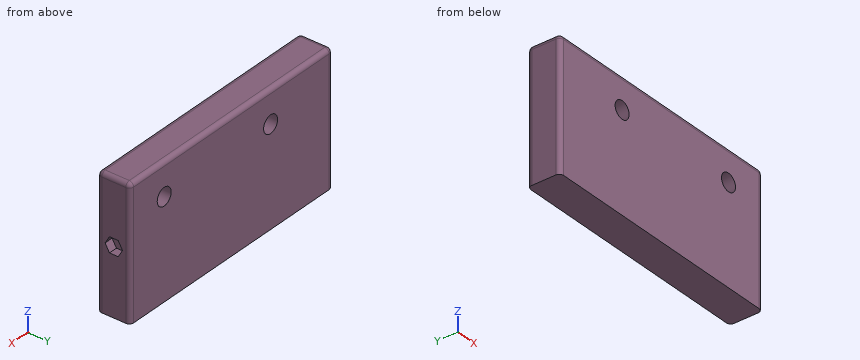
Solid Edge part; units mm, degrees
sketch "Sketch1" plane through (0, 0, 0) normal (1, 0, 0) x (0, 1, 0)
  line L0 (7.5, 30) -> (-7.5, 30)
  line L1 (-7.5, 30) -> (-7.5, -30)
  line L2 (-7.5, -30) -> (7.5, -30)
  line L3 (7.5, -30) -> (7.5, 30)
extrude "largo" add sketch "Sketch1" along normal mid plane 100
hole "Hole1" at (30.5, 7.5, 15) direction (0, -1, 0) diameter 8 end up to next
hole "Hole2" at (-30.5, 7.5, 15) direction (0, -1, 0) diameter 8 end up to next
sketch "Sketch2" plane through (50, -1, -1) normal (1, 0, 0) x (0, 1, 0)
  line L0 (3, 4.9641) -> (-1, 4.9641)
  line L1 (-1, 4.9641) -> (-3, 1.5)
  line L2 (-3, 1.5) -> (-1, -1.9641)
  line L3 (-1, -1.9641) -> (3, -1.9641)
  line L4 (3, -1.9641) -> (5, 1.5)
  line L5 (5, 1.5) -> (3, 4.9641)
extrude "Cutout1" cut sketch "Sketch2" against normal blind 4
sketch "Sketch3" plane through (-50, 0, 0) normal (-1, 0, 0) x (0, -1, 0)
  line L0 (-7.5, -30) -> (-7.5, 30)
  line L1 (-7.5, 30) -> (7.5, 30)
  line L2 (7.5, 30) -> (7.5, -30)
  line L3 (7.5, -30) -> (-7.5, -30)
extrude "ProtrusiónExtruida_5" add sketch "Sketch3" along normal blind 16
fillet "Round1" radius 2 8 edges at (-8, 7.5, 30) (-8, -7.5, 30) (50, 7.5, 0) (50, 0, 30) (-66, -7.5, 0) (-66, 7.5, 0) (-66, 0, 30) (50, -7.5, 0)
Read the model definition and answer for the solid it produces. Units are mm, in the model's axes. Coordinates: 2 decimals unless noted, no trailing zeros. Write each loop counter-clockwise with the first axis right and the second up, starting at its lowest first coordinate (ties: lowest second). Pieces come first, ordered by that corner, then holes. Notation, with made-up numbers: (82, 23.5) -> (122, 23.5) arc R21 cw to (122, 35.5) -> close; hole circle Ø6 at (19, -33). An arc over 180 degrees is marked (long way). Return JSON: item names as keys, results as strings.
(1) This flat-tipped pin is pushed along its axis until it touches: P1, Ø7, axis at x = 30.5, z = 15, coming from the +Y side (1 decimal). Where does it stop, or does it pass through?
Answers below:
{"P1": "through"}
(2) The part is cut by section B-B on x = 30.5. Give the vertices of the cut face in (y, z), then the cut area to 3 significant figures.
Answers below:
{"outline": "(-7.5, -30) -> (7.5, -30) -> (7.5, 11) -> (-7.5, 11) -> close; (-7.5, 19) -> (7.5, 19) -> (7.5, 28) arc R2 ccw to (5.5, 30) -> (-5.5, 30) arc R2 ccw to (-7.5, 28) -> close", "area": "778 mm^2"}
(3) The part is cut by section D-D on z = 2.5. Give the vertices of the cut face in (x, y), then the cut area to 3 significant figures.
Answers below:
{"outline": "(-66, -5.5) arc R2 ccw to (-64, -7.5) -> (48, -7.5) arc R2 ccw to (50, -5.5) -> (50, -2.85) -> (46, -2.85) -> (46, 2.85) -> (50, 2.85) -> (50, 5.5) arc R2 ccw to (48, 7.5) -> (-64, 7.5) arc R2 ccw to (-66, 5.5) -> close", "area": "1,710 mm^2"}
(4) The part is cut by section C-C on x = -28. Give the vertices of the cut face in (y, z).
Answers below:
{"outline": "(-7.5, -30) -> (7.5, -30) -> (7.5, 11.88) -> (-7.5, 11.88) -> close; (-7.5, 18.12) -> (7.5, 18.12) -> (7.5, 28) arc R2 ccw to (5.5, 30) -> (-5.5, 30) arc R2 ccw to (-7.5, 28) -> close"}
(5) The part is cut by section A-A on z = 15. Give the vertices of the cut face in (x, y), then the cut area to 3 significant figures.
Answers below:
{"outline": "(-66, -5.5) arc R2 ccw to (-64, -7.5) -> (-34.5, -7.5) -> (-34.5, 7.5) -> (-64, 7.5) arc R2 ccw to (-66, 5.5) -> close; (-26.5, -7.5) -> (26.5, -7.5) -> (26.5, 7.5) -> (-26.5, 7.5) -> close; (34.5, -7.5) -> (48, -7.5) arc R2 ccw to (50, -5.5) -> (50, 5.5) arc R2 ccw to (48, 7.5) -> (34.5, 7.5) -> close", "area": "1,500 mm^2"}
(6) Consider line 1 along X through (y, z) = (-1, 15); line 2 along Z through (x, y) = (30.5, 2); line 3 along Z through (x, y) = (-34, -4.5). Determine where each line is inside the solid, lowest interval first. Write a range as from..to.
Answers below:
{"line 1": "-66..-34.5, -26.5..26.5, 34.5..50", "line 2": "-30..11, 19..30", "line 3": "-30..13.06, 16.94..30"}
